Read the model definition and answer for the solid it produces. Units are mm, in the model's axes. A direction names the side the tool comes from. Give positions to 0.01 mm unless a question says otherwise; leave off trailing zeros. Order: outer loops, then holes, each group sorted by start corner. A loop starts at its lowest first (then second) coordinate and runs counter-clockwise, first axis right, second up.
```python
from build123d import *

# Parameters (mm, degrees)
F0_W     = 16
F0_H     = 8
F0_W_2   = 14
F0_H_2   = 6
F0_R     = 2.995
F0_R_2   = 2.55
F0_R_3   = 2.4
F1_DEPTH = 1
F2_DEPTH = 1.8
F3_DEPTH = 5
F4_SIZE  = 0.4


# Not quite as in the source:
# - a feature names something its author has since deleted; it is built from what else it names


with BuildPart() as f1:
    # F0 (on Top) → F1 (new body)
    with BuildSketch(Plane.XY):
        Rectangle(F0_W, F0_H)
        Rectangle(F0_W_2, F0_H_2, mode=Mode.SUBTRACT)
        Rectangle(F0_W_2, F0_H_2)
        with Locations((-4, 0)):
            Circle(F0_R, mode=Mode.SUBTRACT)
        with Locations((4, 0)):
            Circle(F0_R, mode=Mode.SUBTRACT)
        with Locations((-4, 0)):
            Circle(F0_R)
        with Locations((-4, 0)):
            Circle(F0_R_2, mode=Mode.SUBTRACT)
        with Locations((4, 0)):
            Circle(F0_R)
        with Locations((4, 0)):
            Circle(F0_R_2, mode=Mode.SUBTRACT)
        with Locations((-4, 0)):
            Circle(F0_R_2)
        with Locations((-4, 0)):
            Circle(F0_R_3, mode=Mode.SUBTRACT)
        with Locations((4, 0)):
            Circle(F0_R_2)
        with Locations((4, 0)):
            Circle(F0_R_3, mode=Mode.SUBTRACT)
        with Locations((4, 0)):
            Circle(F0_R_3)
        with Locations((-4, 0)):
            Circle(F0_R_3)
    extrude(amount=-F1_DEPTH)

    # F0 (on Top) → F2 (join)
    with BuildSketch(Plane.XY):
        with Locations((-4, 0)):
            Circle(F0_R_3)
        with Locations((4, 0)):
            Circle(F0_R_3)
    extrude(amount=F2_DEPTH)

    # F0 (on Top) → F3 (join)
    with BuildSketch(Plane.XY):
        Rectangle(F0_W, F0_H)
        Rectangle(F0_W_2, F0_H_2, mode=Mode.SUBTRACT)
        Rectangle(F0_W_2, F0_H_2)
        with Locations((-4, 0)):
            Circle(F0_R, mode=Mode.SUBTRACT)
        with Locations((4, 0)):
            Circle(F0_R, mode=Mode.SUBTRACT)
        with Locations((4, 0)):
            Circle(F0_R)
        with Locations((4, 0)):
            Circle(F0_R_2, mode=Mode.SUBTRACT)
        with Locations((-4, 0)):
            Circle(F0_R)
        with Locations((-4, 0)):
            Circle(F0_R_2, mode=Mode.SUBTRACT)
    extrude(amount=-F3_DEPTH)

    # F4
    f4_edges = [f1.edges().sort_by_distance(p)[0] for p in [
        (-6.4, 0, 1.8),
        (1.6, 0, 1.8),
        (-8, -4, -2.5),
        (0, -4, -5),
        (8, -4, -2.5),
        (0, -4, 0),
        (-8, 4, -2.5),
        (-8, 0, -5),
        (-8, 0, 0),
        (8, 4, -2.5),
        (0, 4, -5),
        (0, 4, 0),
        (8, 0, -5),
        (8, 0, 0),
        (1.45, 0, -5),
        (-6.55, 0, -5),
    ]]
    chamfer(f4_edges, length=F4_SIZE)


solid = f1.part
```
1) For a pull along Y with two mould halves and no side action, classify faces 4 (the face through (0, 4, -2)), 5 (the face through (-1.644, -0.977, -2.775)), 6 (the face through (-1.71, 0.72, 0.69)), 7 (the face through (8, 0, -2)) as released by +Y, released by -Y, zero draft, split by the parting line, or undercut.
Final values:
face 4: released by +Y
face 5: undercut
face 6: split by the parting line
face 7: zero draft
2) A tool of negligible diameter and unlimited length cuts with its end or side. For faces 1 (the face through (0, -4, -2)), 2 (the face through (-4, 0, -1)), 3 (the face through (6.217, -0.919, 0.69)), from which of +Z, -Z, +X, -X, +Y, -Y can it reach the whole face along a straight path? Write none if from no direction.
Final values:
face 1: +Z, -Z, +X, -X, -Y
face 2: -Z
face 3: +Z
3) Given pin 1 (3 mm diameter, centred on x = 4, y = 0, fed in from -Z), flat-ended and moving along its own axis, determine where the tip first touches the part or whether it passes through.
Final values:
pin 1: stops at z = -1
4) The part is cut by section B-B on z = -2.5. Determine the outline of the cut face in (x, y).
Final values:
outline: (-8, -3.6) - (-7.6, -4) - (7.6, -4) - (8, -3.6) - (8, 3.6) - (7.6, 4) - (-7.6, 4) - (-8, 3.6) - close; hole circle Ø5.1 at (-4, 0); hole circle Ø5.1 at (4, 0)
5) The part is cut by section A-A on x = 4. Determine the outline of the cut face in (y, z), and give its area (3 significant figures).
Final values:
outline: (-4, -4.6) - (-3.6, -5) - (-2.95, -5) - (-2.55, -4.6) - (-2.55, -1) - (2.55, -1) - (2.55, -4.6) - (2.95, -5) - (3.6, -5) - (4, -4.6) - (4, -0.4) - (3.6, 0) - (2.4, 0) - (2.4, 1.4) - (2, 1.8) - (-2, 1.8) - (-2.4, 1.4) - (-2.4, 0) - (-3.6, 0) - (-4, -0.4) - close
area: 27.6 mm2
6) Consider L1, parallel to Y at x = -4, z = -2; L2, parallel to Z at x = 1, y = 2.75; L3, parallel to X at y = -2, z = -3.25. Determine where each line is inside the solid, lowest interval first.
Final values:
L1: y = -4 to -2.55, 2.55 to 4
L2: z = -5 to 0
L3: x = -8 to -5.58, -2.42 to 2.42, 5.58 to 8
